The figure shows three views and two pictorial views of one solid part (mm, origin at its lowest corner). Answer the questions. Coordinates: 2 decimals unless noted, no trailing zeros. Order: outer loops, then holes, each group sorted by start corner. A loop starts at its lowest first (then second) coordinate and runs counter-clockwise, first axis right, second up. Notation, with made-up numbers: M 84.25,-18 L 93.25,-18 A4 ccw 93.25,-13 Z; hole C -15,-12 d1. An arc over 180 degrees is marked long. Use a Markdown table: item, result.
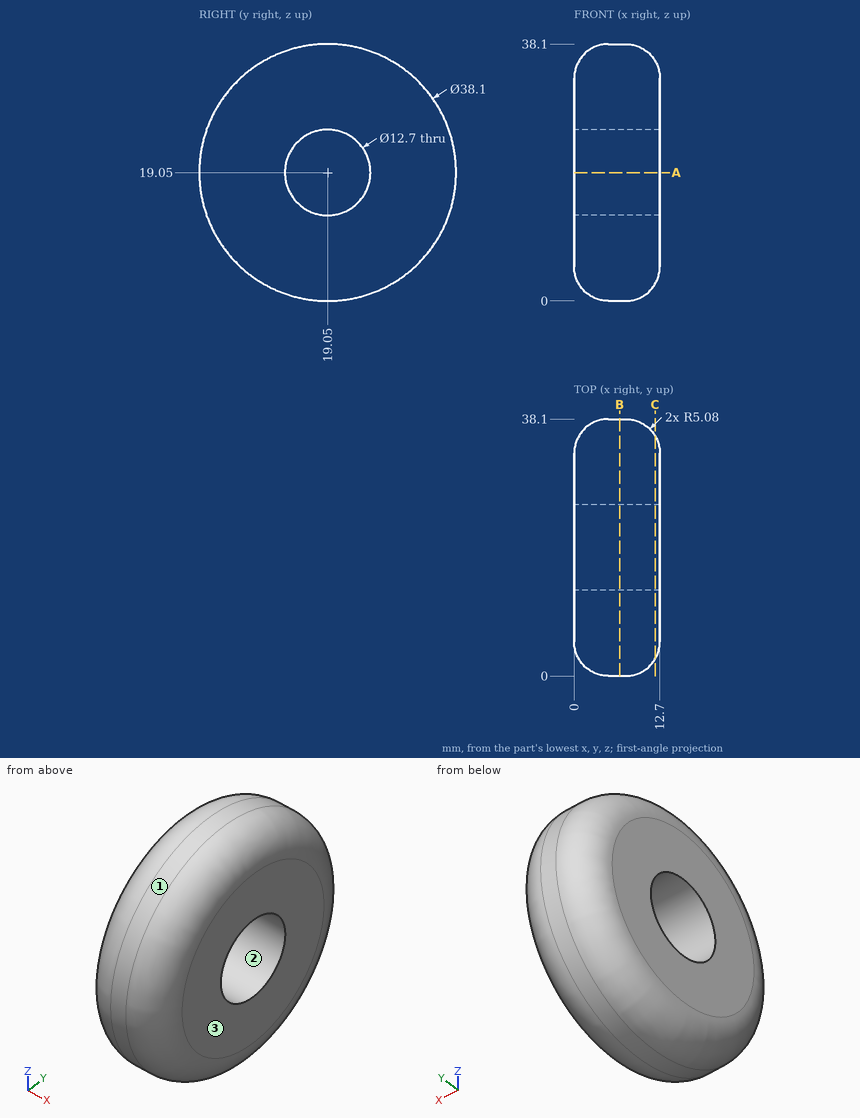
1. Find the intervals of material crossed by probe 1 along Z at (x, y) = (9, 19.05); probe 2 along Z at (x, y) = (7, 19.05); probe 3 along Y at (x, z) = (12, 19.5), in increasing order.
Answers below:
| item | result |
|---|---|
| probe 1 | 0.19 to 12.7, 25.4 to 37.91 |
| probe 2 | 0 to 12.7, 25.4 to 38.1 |
| probe 3 | 2.51 to 12.72, 25.38 to 35.59 |
2. Flat-ended cylindrical pins translate along their axes: P1, Ø3, axis at y = 26.5, z = 7, coming from the +X side; P2, Ø2, axis at x = 5, z = 28, coming from the -Y side; P3, Ø3, axis at x = 3.5, z = 22.5, coming from the -Y side; P4, Ø3, axis at x = 10.5, z = 33.5, coming from the +Y side. Find the tip coordinate at first contact, or state that the pin passes through.
Answers below:
| item | result |
|---|---|
| P1 | x = 12.7 |
| P2 | y = 1.74 |
| P3 | y = 0.18 |
| P4 | y = 32.18 |
3. Section C-C on x = 12 is taken. Determine the outline of the cut face in (y, z), then the cut area to 3 significant figures.
Answers below:
| item | result |
|---|---|
| outline | C 19.05,19.05 d33.09; hole C 19.05,19.05 d12.7 |
| area | 733 mm² |
4. For a pull along Z with two mould halves and no side action, classify the marked faces 1, 2 and 3 as +Z half, -Z half, draft (parallel to the pull), parting line (faces both ways), or undercut.
Answers below:
| item | result |
|---|---|
| face 1 | parting line |
| face 2 | undercut |
| face 3 | draft |
5. Section B-B on x = 6.75 is taken. Determine the outline of the cut face in (y, z), then the cut area to 3 significant figures.
Answers below:
| item | result |
|---|---|
| outline | C 19.05,19.05 d38.1; hole C 19.05,19.05 d12.7 |
| area | 1,010 mm² |
6. Section A-A on z = 19.05 is taken. Determine the outline of the cut face in (x, y).
Answers below:
| item | result |
|---|---|
| outline | M 0,5.08 A5.08 ccw 5.08,0 L 7.62,0 A5.08 ccw 12.7,5.08 L 12.7,12.7 L 0,12.7 Z; M 0,25.4 L 12.7,25.4 L 12.7,33.02 A5.08 ccw 7.62,38.1 L 5.08,38.1 A5.08 ccw 0,33.02 Z |
